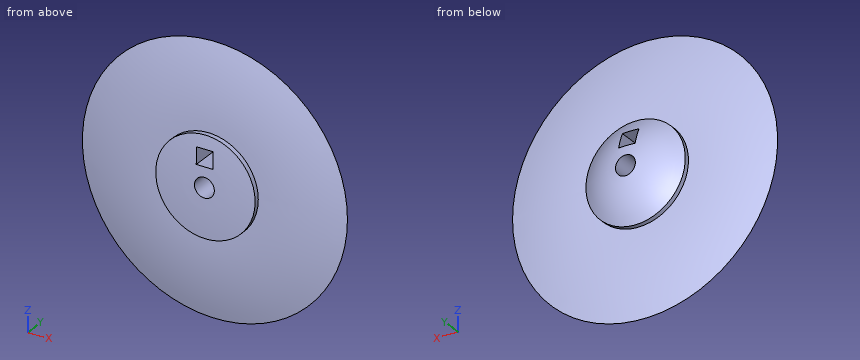
```python
from build123d import *

# Parameters (mm, degrees)
SKETCH2_R          = 3.81
SKETCH2_W          = 6.35
SKETCH2_H          = 6.35
CUT_EXTRUDE1_DEPTH = 20.05


with BuildPart() as part:
    # Sketch1 → Revolve1 (revolve)
    with BuildSketch(Plane.XY):
        with BuildLine():
            Line((0, 0), (0, 19.05))
            ThreePointArc((0, 19.05), (10.040231571, 17.420694713), (19.05, 12.7))
            Line((19.05, 12.7), (19.05, 10.795))
            ThreePointArc((19.05, 10.795), (35.038891456, 9.839095469), (50.8, 6.985))
            ThreePointArc((50.8, 6.985), (35.038891456, 4.130904531), (19.05, 3.175))
            Line((19.05, 3.175), (19.05, 1.27))
            ThreePointArc((19.05, 1.27), (10.801103513, 0.793808666), (2.54, 0.635))
            Line((2.54, 0.635), (2.54, 0))
            Line((2.54, 0), (0, 0))
        make_face()
    revolve(axis=Axis((0, 0, 0), (0, 1, 0)))

    # Sketch2 → Cut-Extrude1 (cut, through all)
    with BuildSketch(Plane.XZ):
        Circle(SKETCH2_R)
        with Locations((0, 10.795)):
            Rectangle(SKETCH2_W, SKETCH2_H)
    extrude(amount=-CUT_EXTRUDE1_DEPTH, mode=Mode.SUBTRACT)

    # Sketch3 → Revolve4 (revolve)
    with BuildSketch(Plane(origin=(0, 5.08, 0), x_dir=(1, 0, 0), z_dir=(0, 1, 0))):
        with BuildLine():
            Line((0, -1.905), (0, -5.715))
            ThreePointArc((0, -5.715), (1.905, -3.81), (0, -1.905))
        make_face()
    revolve(axis=Axis((0, 5.08, 1.905), (0, 0, 1)))


solid = part.part
```
Part model, mm, in its own coordinate system. Coordinates: 2 decimals unless noted, no trailing zeros. Put each result on its own line as item: value. Start each with the question number.
(1) Pin check, flat tips, straight feed: pin 1 Ø2 at (x, z) = (6, -38) entering from -Y; pin 2 Ø6 at (x, z) = (-8.5, 14.5) entering from -Y; pin 3 Ø10 at (x, y) = (-14, 11) entering from +Z. Stop position of each tip, or through.
(2) Band-saw the part on A-A (x = 0). Count the separate pieces of the cut face and the enclosed holes in it, then the cut area to 3 significant figures.
(3) Probe line 1 along Y through (x, z) = (-23.5, -31.5); line 2 along Y through (x, z) = (-26.5, 33); line 3 along X through (y, z) = (11.5, -8). List the from-to ranges inside material, lowest first. Write a range as [from, to].
Determined:
1. pin 1: stops at y = 4.45
1. pin 2: stops at y = 0.93
1. pin 3: stops at z = 49.59
2. separate pieces: 3
2. enclosed holes: 0
2. area: 704 mm²
3. line 1: y = [4.71, 9.26]
3. line 2: y = [5.21, 8.76]
3. line 3: x = [-17.29, 17.29]
